from build123d import *

# Parameters (mm, degrees)
SKETCH1_5_R              = 1.6
BOSS_EXTRUDE1_DEPTH      = 2
BOSS_EXTRUDE1_DEPTH_BACK = 3


with BuildPart() as part:
    # Sketch1 → Revolve2 (revolve)
    with BuildSketch(Plane(origin=(0, 0, 0), x_dir=(1, 0, 0), z_dir=(0, 1, 0))):
        with BuildLine():
            Line((-5, -1.5), (-5, -2))
            Line((-5, -2), (-2.236067977, -2))
            ThreePointArc((-2.236067977, -2), (-2.802517077, -1.070466269), (-3, 0))
            Line((-3, 0), (-9, 0))
            Line((-9, 0), (-9, -1.5))
            Line((-9, -1.5), (-5, -1.5))
        make_face()
        with BuildLine():
            ThreePointArc((-3, 0), (-2.802517077, -1.070466269), (-2.236067977, -2))
            Line((-2.236067977, -2), (-2.236067977, 0))
            Line((-2.236067977, 0), (-3, 0))
        make_face()
        with BuildLine():
            ThreePointArc((3, 0), (2.802517077, -1.070466269), (2.236067977, -2))
            Line((2.236067977, -2), (5, -2))
            Line((5, -2), (5, -1.5))
            Line((5, -1.5), (9, -1.5))
            Line((9, -1.5), (9, 0))
            Line((9, 0), (3, 0))
        make_face()
        with BuildLine():
            Line((2.236067977, 0), (2.236067977, -2))
            ThreePointArc((2.236067977, -2), (2.802517077, -1.070466269), (3, 0))
            Line((3, 0), (2.236067977, 0))
        make_face()
    revolve(axis=Axis((-9, 0, 0), (1, 0, 0)))

    # Sketch1_5 → Boss-Extrude1 (add, two sides)
    with BuildSketch(Plane(origin=(0, 0, 0), x_dir=(1, 0, 0), z_dir=(0, 1, 0))) as boss_extrude1_sk:
        with BuildLine():
            Line((-2.236067977, 0), (-2.236067977, -2))
            ThreePointArc((-2.236067977, -2), (0, -3), (2.236067977, -2))
            Line((2.236067977, -2), (2.236067977, 0))
            Line((2.236067977, 0), (3, 0))
            ThreePointArc((3, 0), (2.802517077, 1.070466269), (2.236067977, 2))
            ThreePointArc((2.236067977, 2), (0, 3), (-2.236067977, 2))
            ThreePointArc((-2.236067977, 2), (-2.802517077, 1.070466269), (-3, 0))
            Line((-3, 0), (-2.236067977, 0))
        make_face()
        Circle(SKETCH1_5_R, mode=Mode.SUBTRACT)
        with BuildLine():
            Line((2.236067977, 0), (2.236067977, -2))
            ThreePointArc((2.236067977, -2), (2.802517077, -1.070466269), (3, 0))
            Line((3, 0), (2.236067977, 0))
        make_face()
        with BuildLine():
            ThreePointArc((-3, 0), (-2.802517077, -1.070466269), (-2.236067977, -2))
            Line((-2.236067977, -2), (-2.236067977, 0))
            Line((-2.236067977, 0), (-3, 0))
        make_face()
    extrude(amount=BOSS_EXTRUDE1_DEPTH)
    extrude(boss_extrude1_sk.sketch, amount=-BOSS_EXTRUDE1_DEPTH_BACK)


solid = part.part
Geometry check sheet. Reference: the model listing, model coordinates, mm. A direction names the side the tool comes from. Give positions to 0.01 mm unless a question says otherwise; leave off trailing zeros. Loops run counter-clockwise (first coordinate to the right, second up) from the corner with the lowest first, then second, coordinate; pieces in that order, holes last. Notation, with made-up numbers: M 70,-34.75 L 92,-34.75 A31 ccw 92,3.25 Z; hole C -2,-17 d9. An arc over 180 degrees is marked long. Answer as a JSON object with one key per item and string values. Group by question number.
Item 1: Sectioned sample at A-A on x = 0. Record the boundary of the cut face in (y, z), plus the area to 3 significant figures.
Item 2: Sectioned sample at D-D on x = 2. Record the boundary of the cut face in (y, z).
Item 3: Sectioned sample at C-C on z = -1.25. Record the boundary of the cut face in (x, y).
Item 4: Material ranges on L1, parallel to Z at x = 0, y = -1.2; L2, parallel to X at y = 0.5, z = 0; L3, parallel to X at y = 0.9, z = -0.75, recorded low to high.
Item 5: Access from +Z, -Z, +X, -X, +Y, -Y to the whole of each face (thin tool, end or side, straight path). Record for faces 1 (the cylindrical face through (3.944, 0.766, 1.847)), 2 (the cylindrical face through (-3.906, 1.774, 0.923)), 3 (the flat face through (-9, 0, 0)).
Item 6: Sectioned sample at B-B on y = 0.55. Record the boundary of the cut face in (x, z), plus the area to 3 significant figures.
Item 7: Gauge pin test, flat ends, axial feed: pin 1 (2 mm diameter, centred on x = -4, z = -2, fed in from -Y); pin 2 (1.5 mm diameter, centred on x = -7, y = 1.5, fed in from -Z); pin 3 (1 mm diameter, centred on x = -1.5, y = 0.5, fed in from +Z). Record the tip position at first contact, or that the pin passes through.
Findings below:
{
 "1": {"outline": "M -3,-3 L 2,-3 L 2,-1.6 L -3,-1.6 Z; M -3,1.6 L 2,1.6 L 2,3 L -3,3 Z", "area": "14.0 mm2"},
 "2": {"outline": "M -3,-2.24 L 2,-2.24 L 2,2.24 L -3,2.24 Z"},
 "3": {"outline": "M -9,-0.83 L -5,-0.83 L -5,-1.56 L -2.73,-1.56 L -2.73,-3 L -1,-3 L -1,2 L -2.73,2 L -2.73,1.56 L -5,1.56 L -5,0.83 L -9,0.83 Z; M 1,-3 L 2.73,-3 L 2.73,-1.56 L 5,-1.56 L 5,-0.83 L 9,-0.83 L 9,0.83 L 5,0.83 L 5,1.56 L 2.73,1.56 L 2.73,2 L 1,2 Z"},
 "4": {"L1": "-3 to -1.6, 1.6 to 3", "L2": "-9 to -1.6, 1.6 to 9", "L3": "-9 to -1.41, 1.41 to 9"},
 "5": {"face 1": "+X", "face 2": "-X", "face 3": "+Z, -Z, -X, +Y, -Y"},
 "6": {"outline": "M -9,-1.4 L -5,-1.4 L -5,-1.92 L -2.3,-1.92 A3 ccw 2.3,-1.92 L 5,-1.92 L 5,-1.4 L 9,-1.4 L 9,1.4 L 5,1.4 L 5,1.92 L 2.3,1.92 A3 ccw -2.3,1.92 L -5,1.92 L -5,1.4 L -9,1.4 Z; hole C 0,0 d3.2", "area": "59.6 mm2"},
 "7": {"pin 1": "y = -1.73", "pin 2": "z = -1.3", "pin 3": "z = 2.83"}
}
